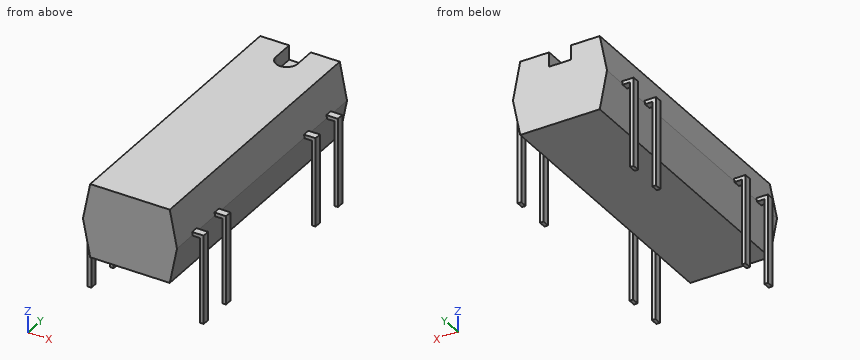
from build123d import *

# Parameters (mm, degrees)
PAD003_DEPTH = 0.25
PAD_DEPTH    = 9.65
POCKET_DEPTH = 1
PAD002_DEPTH = 0.25
PAD001_DEPTH = 0.25
PAD004_DEPTH = 0.25


with BuildPart() as pad003:
    # Sketch004 → Pad003 (new body, symmetric)
    with BuildSketch(Plane.XZ.offset(2.54)):
        Polygon((-0.2, -3.2), (0.05, -3.2), (0.05, 2.7), (7.57, 2.7), (7.57, -3.2), (7.82, -3.2), (7.82, 2.95), (-0.2, 2.95), align=None)
    extrude(amount=PAD003_DEPTH, both=True)


with BuildPart() as pocket:
    # Sketch → Pad (new body, symmetric)
    with BuildSketch(Plane.XZ.offset(7.62)):
        Polygon((1.06, 0.2), (6.56, 0.2), (7.06, 2.75), (6.56, 5.3), (1.06, 5.3), (0.56, 2.75), align=None)
    extrude(amount=PAD_DEPTH, both=True)

    # Sketch003 → Pocket (cut)
    with BuildSketch(Plane(origin=(0, -7.62, 5.3), x_dir=(-1, 0, 0), z_dir=(0, 0, 1))):
        with BuildLine():
            ThreePointArc((-3.06, -8.15), (-3.81, -7.4), (-4.56, -8.15))
            Line((-4.56, -8.15), (-4.56, -9.65))
            Line((-4.56, -9.65), (-3.06, -9.65))
            Line((-3.06, -9.65), (-3.06, -8.15))
        make_face()
    extrude(amount=-POCKET_DEPTH, mode=Mode.SUBTRACT)


with BuildPart() as pad002:
    # Sketch002 → Pad002 (new body, symmetric)
    with BuildSketch(Plane.XZ.offset(15.24)):
        Polygon((-0.2, -3.2), (0.05, -3.2), (0.05, 2.7), (7.57, 2.7), (7.57, -3.2), (7.82, -3.2), (7.82, 2.95), (-0.2, 2.95), align=None)
    extrude(amount=PAD002_DEPTH, both=True)


with BuildPart() as pad001:
    # Sketch001 → Pad001 (new body, symmetric)
    with BuildSketch(Plane.XZ):
        Polygon((-0.2, -3.2), (0.05, -3.2), (0.05, 2.7), (7.57, 2.7), (7.57, -3.2), (7.82, -3.2), (7.82, 2.95), (-0.2, 2.95), align=None)
    extrude(amount=PAD001_DEPTH, both=True)


with BuildPart() as obj1:
    # Sketch005 → Pad004 (new body, symmetric)
    with BuildSketch(Plane.XZ.offset(12.7)):
        Polygon((-0.2, -3.2), (0.05, -3.2), (0.05, 2.7), (7.57, 2.7), (7.57, -3.2), (7.82, -3.2), (7.82, 2.95), (-0.2, 2.95), align=None)
    extrude(amount=PAD004_DEPTH, both=True)

    add(pad003.part)
    add(pocket.part)
    add(pad002.part)
    add(pad001.part)


solid = obj1.part
Read the model definition and answer for the solid it produces. Units are mm, in the model's axes. Give positions to 0.01 mm unless a question says otherwise; leave off trailing zeros. Write each loop counter-clockwise with the first axis right and the second up, starting at its lowest first coordinate (ties: lowest second). Pieces come first, ordered by that corner, then holes. Notation, with made-up numbers: (-1, 55) - (24, 55) arc R16 ccw to (24, 73) - close; hole circle Ø8 at (-34, 24.25). An arc over 180 degrees is marked (long way). Return JSON: item names as keys, results as strings.
Q1. A cutting plane is placed at A-A, the plane z = -0.75. Count the separate pieces of the cut face and the enclosed holes in it, and give its area (3 significant figures).
Reply:
{"separate pieces": "8", "enclosed holes": "0", "area": "1.00 mm²"}
Q2. A cutting plane is placed at C-C, the plane y = -6.5. Determine the outline of the cut face in (x, z), and give its area (3 significant figures).
Reply:
{"outline": "(0.56, 2.75) - (1.06, 0.2) - (6.56, 0.2) - (7.06, 2.75) - (6.56, 5.3) - (1.06, 5.3) - close", "area": "30.6 mm²"}
Q3. Given P1, Ø0.9, axis at x = 7.5, z = -1.5, coming from the +Y side; P2, Ø0.6, axis at x = 7.5, y = -13, coming from the +Z side; P3, Ø3, axis at x = 3.5, y = -9.5, coming from the -Z side; P4, Ø3, axis at x = 3, z = -2, coming from the -Y side, each flat-ended and moving along its own axis, determine where each tip first touches the part or whether it passes through.
Reply:
{"P1": "y = 0.25", "P2": "z = 2.95", "P3": "z = 0.2", "P4": "through"}
Q4. A cutting plane is placed at B-B, the plane x = 3.81. Determine the outline of the cut face in (y, z), and give its area (3 significant figures).
Reply:
{"outline": "(-17.27, 0.2) - (2.03, 0.2) - (2.03, 4.3) - (-0.22, 4.3) - (-0.22, 5.3) - (-17.27, 5.3) - close", "area": "96.2 mm²"}
Q5. Consider line 1 along X through (y, z) = (-2.75, -0.25); line 2 along Z through (x, y) = (2, -4.5); line 3 along X through (y, z) = (-16.5, 2.75). Determine where each line is inside the solid, lowest interval first. Write a range as [from, to].
Reply:
{"line 1": "[-0.2, 0.05], [7.57, 7.82]", "line 2": "[0.2, 5.3]", "line 3": "[0.56, 7.06]"}
